Autodesk Inventor part; units mm, degrees
ref_plane "YZ Plane" through (0, 0, 0) normal (1, 0, 0) x (0, 1, 0)
ref_plane "XZ Plane" through (0, 0, 0) normal (0, 1, 0) x (-1, 0, 0)
ref_plane "XY Plane" through (0, 0, 0) normal (0, 0, 1) x (1, 0, 0)
sketch "Sketch1" plane through (0, 0, 0) normal (0, 0, 1) x (1, 0, 0)
  circle A0 centre (0, 19.7) radius 2.1828
  circle A1 centre (0, -19.7) radius 2.1828
  line L0 (-6.35, -26.05) -> (6.35, -26.05)
  line L1 (6.35, -26.05) -> (6.35, 26.05)
  line L2 (6.35, 26.05) -> (-6.35, 26.05)
  line L3 (-6.35, 26.05) -> (-6.35, -26.05)
  line L4 (-6.35, -26.05) -> (6.35, 26.05) construction
  line L5 (6.35, -26.05) -> (-6.35, 26.05) construction
  point P0 (0, 0)
  dimension "d0" = 4.3656
  dimension "d1" = 4.3656
  dimension "d2" = 19.7
  dimension "d3" = 39.4
  dimension "d4" = 12.7
  dimension "d5" = 6.35
  dimension "d6" = 6.35
  dimension "d7" = 6.35
extrude "Extrusion1" add sketch "Sketch1" along normal blind 1.5875
fillet "Fillet1" radius 0.7937 4 edges at (-6.35, 0, 0) (-6.35, 0, 1.5875) (6.35, 0, 0) (6.35, 0, 1.5875)
properties part number "Part F"
For this review, take the finished solid that the model builds, in its own axes (mm). Round coordinates to 2 decimals unless told otherwise and drop trailing zeros. Loops run counter-clockwise (first coordinate to the right, second up) from the corner with the lowest first, then second, coordinate; pieces in that order, holes last.
(1) We need section D-D (z = 1.1). Give the boundary of the cut face in (x, y).
Returned:
outline: (-6.29, -26.05) - (6.29, -26.05) - (6.29, 26.05) - (-6.29, 26.05) - close; hole circle Ø4.37 at (0, -19.7); hole circle Ø4.37 at (0, 19.7)
(2) We need section A-A (x = 0). Give the boundary of the cut face in (y, z), plus the area to 3 significant figures.
Returned:
outline: (-26.05, 0) - (-21.88, 0) - (-21.88, 1.59) - (-26.05, 1.59) - close; (-17.52, 0) - (17.52, 0) - (17.52, 1.59) - (-17.52, 1.59) - close; (21.88, 0) - (26.05, 0) - (26.05, 1.59) - (21.88, 1.59) - close
area: 68.8 mm2
(3) Mouldability with a two-part tool opening along Y and no side actions: class faces 1 (the flat face through (0, -26.05, 1)), 2 (the flat face through (0, 0, 1.588)), 3 (the flat face through (0, 26.05, 1)), 4 (the cylindrical face through (-0.284, -21.864, 0.783)) as released by +Y, released by -Y, zero draft, split by the parting line, or undercut.
Returned:
face 1: released by -Y
face 2: zero draft
face 3: released by +Y
face 4: undercut
(4) Wall thickness on line 1 along Y through (x, z) = (0, 0.55); line 2 along X through (y, z) = (9.5, 0.9); line 3 along X through (y, z) = (-13, 1.25): over which ranges is each line inside the solid? List them lowest first.
Returned:
line 1: y = -26.05 to -21.88, -17.52 to 17.52, 21.88 to 26.05
line 2: x = -6.34 to 6.34
line 3: x = -6.21 to 6.21
(5) Clearance check with a flat-ended pin moving along its axis: P1, Ø5.5, axis at x = 0, y = 19.7, coming from the -Z side. State where the tip first meets the part, or that it passes through.
Returned:
P1: stops at z = 0
